For this review, take the finished solid that the model builds, in its own axes (mm). Face numbers are marked on the shaded views. A direction names the side the tool comes from. Round coordinates to 2 decimals unless told otherwise and drop trailing zeros. Loops run counter-clockwise (first coordinate to the right, second up) from the corner with the lowest first, then second, coordinate; pieces in that order, holes last.
1. Tool access review of the marked faces 1, 2 and 3: name each direction out of +Z, -Z, +X, -X, +Y, -Y from which nothing blocks a thin tool from reaching the whole face with its end or side.
2. Draft analysis for pull direction Y (two halves, no side actions). For the marked faces 4 and 5, state which applies: released by +Y, released by -Y, zero draft, split by the parting line, or undercut.
3. Consider section C-C on x = 2.75. State the section outline as (y, z) points.
4. Consider section D-D on y = -6.5. State the section outline as (x, z) points.
5. Consider section A-A on z = 3.75. State the section outline as (x, y) points.
6. Consider section B-B on x = 0. State the section outline as (y, z) points.
7. To check wall thickness, follow line 1 along Y through (x, z) = (0, -0.4); line 2 along X through (y, z) = (0, -0.3); line 3 along Z through (x, y) = (2.5, -6.5). State the ranges of each line that lie inside material, in increasing order.
8. Clearance check with flat-ended pins moving along their axes: pin 1 Ø4 at (x, z) = (-6, 1.5) entering from -Y; pin 2 Ø1 at (x, y) = (-3.5, 2.5) entering from +Z; pin 3 Ø3 at (y, z) = (2.5, 4) entering from -X. State where each tip first meets the part, or that it passes through.
from build123d import *

# Parameters (mm, degrees)
BOSS_EXTRUDE1_DEPTH = 6
BOSS_EXTRUDE2_START = 1
BOSS_EXTRUDE2_DEPTH = 1
CUT_EXTRUDE1_START  = -6
CUT_EXTRUDE1_DEPTH  = 6
CUT_EXTRUDE2_START  = -6
CUT_EXTRUDE2_DEPTH  = 6
FILLET1_R           = 1.2


with BuildPart() as part:
    # Sketch1 → Boss-Extrude1 (new body)
    with BuildSketch(Plane.XY):
        with BuildLine():
            Line((3.987754263, 1.859520352), (5.437846722, 2.53570957))
            ThreePointArc((5.437846722, 2.53570957), (-6, 0), (5.437846722, -2.53570957))
            Line((5.437846722, -2.53570957), (3.987754263, -1.859520352))
            ThreePointArc((3.987754263, -1.859520352), (-4.4, 0), (3.987754263, 1.859520352))
        make_face()
    extrude(amount=BOSS_EXTRUDE1_DEPTH)

    # Sketch2 → Boss-Extrude2 (add)
    with BuildSketch(Plane(origin=(0, 0, 0), x_dir=(-1, 0, 0), z_dir=(0, 0, -1)).offset(BOSS_EXTRUDE2_START)):
        with BuildLine():
            Line((-3.987754263, -1.859520352), (-5.437846722, -2.53570957))
            ThreePointArc((-5.437846722, -2.53570957), (6, 0), (-5.437846722, 2.53570957))
            Line((-5.437846722, 2.53570957), (-3.987754263, 1.859520352))
            ThreePointArc((-3.987754263, 1.859520352), (4.4, 0), (-3.987754263, -1.859520352))
        make_face()
        with BuildLine():
            Line((-6.797308403, 3.169636963), (-5.437846722, 2.53570957))
            ThreePointArc((-5.437846722, 2.53570957), (6, 0), (-5.437846722, -2.53570957))
            Line((-5.437846722, -2.53570957), (-6.797308403, -3.169636963))
            ThreePointArc((-6.797308403, -3.169636963), (1.623297105, -7.322220053), (7.5, 0))
            ThreePointArc((7.5, 0), (1.623297105, 7.322220053), (-6.797308403, 3.169636963))
        make_face()
    extrude(amount=-BOSS_EXTRUDE2_DEPTH)

    # Sketch3 → Cut-Extrude1 (cut)
    with BuildSketch(Plane.XY.offset(6).offset(CUT_EXTRUDE1_START)):
        with BuildLine():
            ThreePointArc((-5.503902596, -2.388944581), (-4.914912266, -3.441458618), (-4.127319149, -4.354909487))
            Line((-4.127319149, -4.354909487), (-2.779344429, -3.411047427))
            ThreePointArc((-2.779344429, -3.411047427), (-3.604268995, -2.52373632), (-4.155927876, -1.44508252))
            Line((-4.155927876, -1.44508252), (-5.503902596, -2.388944581))
        make_face()
        with BuildLine():
            ThreePointArc((-5.376200178, 5.229385398), (-6.143640332, 4.301823273), (-6.752783625, 3.263420492))
            Line((-6.752783625, 3.263420492), (-5.503902596, 2.388944581))
            ThreePointArc((-5.503902596, 2.388944581), (-4.914912266, 3.441458618), (-4.127319149, 4.354909487))
            Line((-4.127319149, 4.354909487), (-5.376200178, 5.229385398))
        make_face()
        with BuildLine():
            ThreePointArc((-4.127319149, 4.354909487), (-4.914912266, 3.441458618), (-5.503902596, 2.388944581))
            Line((-5.503902596, 2.388944581), (-4.155927876, 1.44508252))
            ThreePointArc((-4.155927876, 1.44508252), (-3.604268995, 2.52373632), (-2.779344429, 3.411047427))
            Line((-2.779344429, 3.411047427), (-4.127319149, 4.354909487))
        make_face()
        with BuildLine():
            ThreePointArc((-6.752783625, -3.263420492), (-6.143640332, -4.301823273), (-5.376200178, -5.229385398))
            Line((-5.376200178, -5.229385398), (-4.127319149, -4.354909487))
            ThreePointArc((-4.127319149, -4.354909487), (-4.914912266, -3.441458618), (-5.503902596, -2.388944581))
            Line((-5.503902596, -2.388944581), (-6.752783625, -3.263420492))
        make_face()
    extrude(amount=CUT_EXTRUDE1_DEPTH, mode=Mode.SUBTRACT)

    # Sketch4 → Cut-Extrude2 (cut)
    with BuildSketch(Plane.XY.offset(6).offset(CUT_EXTRUDE2_START)):
        with BuildLine():
            Line((-4.155927876, 1.44508252), (-5.503902596, 2.388944581))
            ThreePointArc((-5.503902596, 2.388944581), (-6, 0), (-5.503902596, -2.388944581))
            Line((-5.503902596, -2.388944581), (-4.155927876, -1.44508252))
            ThreePointArc((-4.155927876, -1.44508252), (-4.4, 0), (-4.155927876, 1.44508252))
        make_face()
    extrude(amount=CUT_EXTRUDE2_DEPTH, mode=Mode.SUBTRACT)

    # Fillet1
    # the kernel refuses this fillet: 1.2 mm, written as the material it adds along each edge
    with BuildSketch(Plane(origin=(-0.321888296, 1.690318118, 0), x_dir=(0, 0, 1), z_dir=(-0.8191520442889906, 0.5735764363510478, 0))) as fillet1_piece_1_section:
        with BuildLine():
            CenterArc((FILLET1_R, -FILLET1_R), FILLET1_R, 90, 90)
            Line((0, -FILLET1_R), (0, 0))
            Line((0, 0), (FILLET1_R, 0))
        make_face()
    fillet1_piece_1 = extrude(amount=7.645573285, mode=Mode.PRIVATE)
    fillet1_piece_1 = fillet1_piece_1 - Plane(origin=(0, 0, 0.272987798), x_dir=(0.9063077870366507, -0.4226182617406978, 0), z_dir=(0, 0, -1)) * Cylinder(4.4, 21, mode=Mode.PRIVATE)
    fillet1_piece_1 = fillet1_piece_1 & Plane(origin=(0, 0, 0.272987798), x_dir=(0.9063077870366507, 0.4226182617406977, 0), z_dir=(0, 0, -1)) * Cylinder(6, 21, mode=Mode.PRIVATE)
    with BuildSketch(Plane(origin=(-6.584775282, -6.075638796, 0), x_dir=(-0.5735764363510464, 0.8191520442889915, 0), z_dir=(0.8191520442889916, 0.5735764363510465, 0))) as fillet1_piece_2_section:
        with BuildLine():
            CenterArc((FILLET1_R, FILLET1_R), FILLET1_R, 180, 90)
            Line((0, FILLET1_R), (0, 0))
            Line((0, 0), (FILLET1_R, 0))
        make_face()
    fillet1_piece_2 = extrude(amount=7.645573285, mode=Mode.PRIVATE)
    fillet1_piece_2 = fillet1_piece_2 - Plane(origin=(0, 0, 0.272987172), x_dir=(0.9063077870366507, 0.4226182617406977, 0), z_dir=(0, 0, -1)) * Cylinder(4.4, 21, mode=Mode.PRIVATE)
    fillet1_piece_2 = fillet1_piece_2 & Plane(origin=(0, 0, 0.272987172), x_dir=(0.9063077870366507, 0.4226182617406977, 0), z_dir=(0, 0, -1)) * Cylinder(6, 21, mode=Mode.PRIVATE)
    add([fillet1_piece_1, fillet1_piece_2])


solid = part.part
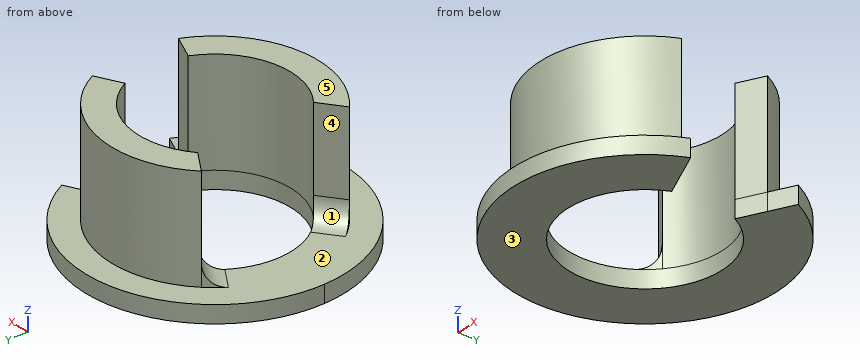
Resolved:
1. face 1: +Z, -X
1. face 2: +Z
1. face 3: -Z, +X, -X, +Y, -Y
2. face 4: undercut
2. face 5: zero draft
3. outline: (-6.98, -1) - (-3.43, -1) - (-3.43, 6) - (-5.33, 6) - (-5.33, 0) - (-6.98, 0) - close; (3.43, -1) - (6.98, -1) - (6.98, 0) - (5.33, 0) - (5.33, 6) - (3.43, 6) - close
4. outline: (-3.74, -1) - (3.74, -1) - (3.74, 0) - (-3.74, 0) - close
5. outline: (-4.13, -4.35) arc R6 ccw to (5.44, -2.54) - (3.99, -1.86) arc R4.4 cw to (-2.78, -3.41) - close; (-4.13, 4.35) - (-2.78, 3.41) arc R4.4 cw to (3.99, 1.86) - (5.44, 2.54) arc R6 ccw to start
6. outline: (-7.5, -1) - (-4.4, -1) - (-4.4, 6) - (-6, 6) - (-6, 0) - (-7.5, 0) - close; (4.4, -1) - (7.5, -1) - (7.5, 0) - (6, 0) - (6, 6) - (4.4, 6) - close
7. line 1: y = -7.5 to -4.4, 4.4 to 7.5
7. line 2: x = -7.5 to -4.4
7. line 3: z = -1 to 0
8. pin 1: stops at y = -5.86
8. pin 2: stops at z = 0.13
8. pin 3: stops at x = -3.62
